Autodesk Inventor part; units mm, degrees
ref_plane "P3_XY" through (0, 0, 0) normal (0, 0, -1) x (1, 0, 0)
ref_plane "P3_YZ" through (0, 0, 0) normal (1, 0, 0) x (0, -1, 0)
ref_plane "P3_ZX" through (0, 0, 0) normal (0, -1, 0) x (0, 0, -1)
sketch "Sketch_1" plane through (0, 0, 0) normal (1, 0, 0) x (0, 0, -1)
  line L0 (0, 12.3912) -> (0, -11.05)
  line L1 (0, -11.05) -> (1, -11.05)
  line L2 (1, -11.05) -> (1, 12.4)
  line L3 (1, 12.4) -> (5.6693, 12.4)
  arc A0 (6.1684, 11.8695) -> (5.6693, 12.4) centre (5.6693, 11.9) ccw
  line L4 (6.1684, 11.8695) -> (4.8747, -9.2828)
  arc A1 (4.8747, -9.2828) -> (5.3282, -10.1825) centre (5.8728, -9.3439) ccw
  line L5 (5.3282, -10.1825) -> (7.9554, -11.8887)
  line L6 (7.9554, -11.8887) -> (8.5, -11.05)
  line L7 (8.5, -11.05) -> (6.1173, -9.5027)
  arc A2 (5.8906, -9.0528) -> (6.1173, -9.5027) centre (6.3897, -9.0834) ccw
  line L8 (5.8906, -9.0528) -> (7.1957, 12.2848)
  arc A3 (7.1957, 12.2848) -> (6.2063, 13.3458) centre (6.1975, 12.3459) ccw
  line L9 (6.2063, 13.3458) -> (1.0087, 13.3912)
  arc A4 (1.0087, 13.3912) -> (0, 12.3912) centre (1, 12.3912) ccw
extrude "Extrusion1" add sketch "Sketch_1" along normal mid plane 18
sketch "Sketch_2" plane through (0, 0, 0) normal (0, 0, 1) x (1, 0, 0)
  line L0 (-6.75, 16.5) -> (-6.75, 12.5)
  arc A0 (-6.75, 12.5) -> (-5.75, 11.5) centre (-5.75, 12.5) ccw
  line L1 (-5.75, 11.5) -> (5.75, 11.5)
  arc A1 (5.75, 11.5) -> (6.75, 12.5) centre (5.75, 12.5) ccw
  line L2 (6.75, 12.5) -> (6.75, 16.5)
  line L3 (6.75, 16.5) -> (-6.75, 16.5)
extrude "Extrusion2" cut sketch "Sketch_2" against normal blind 8
sketch "Sketch_3" plane through (0, 0, -1) normal (0, 0, 1) x (1, 0, 0)
  line L0 (-6.5, -12) -> (6.5, -12)
  line L1 (6.5, -12) -> (6.5, 13)
  line L2 (6.5, 13) -> (-6.5, 13)
  line L3 (-6.5, 13) -> (-6.5, -12)
extrude "Extrusion3" cut sketch "Sketch_3" against normal blind 8
sketch "Sketch_4" plane through (0, 0, 0) normal (1, 0, 0) x (0, 0, -1)
  arc A0 (4, -7.9626) -> (5.1384, -10.0593) centre (6.5, -7.9626) ccw
  line L0 (5.1384, -10.0593) -> (7.9554, -11.8887)
  line L1 (7.9554, -11.8887) -> (8.5, -11.05)
  line L2 (8.5, -11.05) -> (5.4554, -9.0728)
  arc A1 (5, -8.2341) -> (5.4554, -9.0728) centre (6, -8.2341) ccw
  line L3 (5, -8.2341) -> (5, 13.4)
  line L4 (5, 13.4) -> (4, 13.4)
  line L5 (4, 13.4) -> (4, -7.9626)
extrude "Extrusion4" add sketch "Sketch_4" along normal mid plane 13
sketch "Sketch_5" plane through (0, 0, 0) normal (1, 0, 0) x (0, 0, -1)
  line L0 (13, 0) -> (4, 0)
  line L1 (4, 0) -> (4, 5.7)
  line L2 (4, 5.7) -> (5, 5.7)
  arc A0 (5, 5.7) -> (6, 4.7) centre (6, 5.7) ccw
  line L3 (6, 4.7) -> (12, 4.7)
  arc A1 (13, 3.7) -> (12, 4.7) centre (12, 3.7) ccw
  line L4 (13, 3.7) -> (13, 0)
  line L5 (13, 0) -> (4, 0)
revolve "Revolution1" add sketch "Sketch_5" angle 360 about axis through (0, 0, -13) along (0, 0, -1)
sketch "Sketch6" plane through (0, 0, -13) normal (0, 0, -1) x (-1, 0, 0)
  point P0 (0, 0)
hole "Hole1" at (0, 0, -13) direction (0, 0, 1) diameter 7 depth 14
ref_plane "P3_XY" through (0, 0, 0) normal (0, 0, -1) x (1, 0, 0)
ref_plane "P3_YZ" through (0, 0, 0) normal (1, 0, 0) x (0, -1, 0)
ref_plane "P3_ZX" through (0, 0, 0) normal (0, -1, 0) x (0, 0, -1)
properties part number "8617.540_P3"
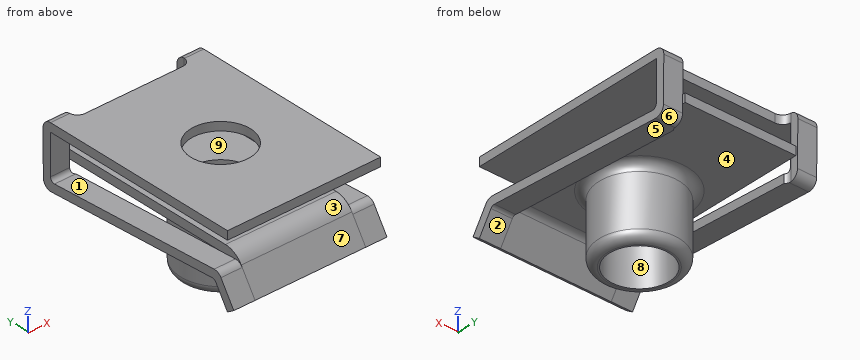
For this review, take the finished solid that the model builds, in its own axes (mm). Face numbers are marked on the shaded views. A direction names the side the tool comes from. Round coordinates to 2 decimals unless told otherwise and drop trailing zeros. Order: outer loops, then holes, each group sorted by start corner. A loop starts at its lowest first (then second) coordinate and runs counter-clockwise, first axis right, second up. Notation, with made-up numbers: M -11.5,12 L 30.5,12 A27 cw 30.5,32 Z; hole C -21.5,-6.5 d8. An arc over 180 degrees is marked long. Use a Markdown table: item, result. Add a question column.
Item 1: Add section D-D, the plane y = 0. State how many separate pieces and enclosed holes the cut face has, then the cut area to 3 significant figures.
Item 2: Add section B-B, the plane y = -6. Give the boundary of the cut face in (x, z).
Item 3: Mouldability with a two-part tool opening along Z and no side actions: class the marked faces 6, 7, 8 and 9 as released by +Z, released by -Z, zero draft, split by the parting line, or undercut.
Item 4: Insertion check: pin 1 (0.7 mm diameter, centred on x = 8, z = -2.5, fed in from -Y); pin 2 (0.8 mm diameter, centred on x = 0, z = -0.5, fed in from +Y); pin 3 (1 mm diameter, centred on y = 4.5, z = -4.5, fed in from -X). Each pin has a flat end and moves straight along its axis. Give the tip position at first contact, or say it passes through.
Item 5: Add section A-A, the plane x = 0. Give the boundary of the cut face in (y, z).
Item 6: To check wall thickness, follow line 1 along X through (y, z) = (0, -6.25); line 2 along X through (y, z) = (0, -0.7); line 3 along Y through (x, z) = (-1.25, -5.75). State the ranges of each line that lie inside material, in increasing order.
Item 7: Tool access review of the marked faces 1, 2, 3, 4 and 5: name each direction out of +Z, -Z, +X, -X, +Y, -Y from which nothing blocks a thin tool from reaching the whole face with its end or side.
Item 8: Add section C-C, the plane z = -11. Give the boundary of the cut face in (x, y).
Geometry results:
| question | item | result |
|---|---|---|
| 1 | separate pieces | 6 |
| 1 | enclosed holes | 0 |
| 1 | area | 41.2 mm² |
| 2 | outline | M -9,-6.08 L -6.5,-6.08 L -6.5,-5.08 L -9,-5.08 Z; M -9,-1 L 9,-1 L 9,0 L -9,0 Z; M -6.5,-5 L 6.5,-5 L 6.5,-4 L -6.5,-4 Z; M 6.5,-6.08 L 9,-6.08 L 9,-5.08 L 6.5,-5.08 Z |
| 3 | face 6 | released by -Z |
| 3 | face 7 | undercut |
| 3 | face 8 | zero draft |
| 3 | face 9 | undercut |
| 4 | pin 1 | stops at y = 12.4 |
| 4 | pin 2 | stops at y = 11.5 |
| 4 | pin 3 | stops at x = -6.5 |
| 5 | outline | M -11.89,-7.96 L -11.05,-8.5 L -9.07,-5.46 A1 cw -8.23,-5 L -5.7,-5 A1 cw -4.7,-6 L -4.7,-12 A1 ccw -3.7,-13 L -3.5,-13 L -3.5,-4 L -7.96,-4 A2.5 ccw -10.06,-5.14 Z; M -11.05,-1 L -3.5,-1 L -3.5,0 L -11.05,0 Z; M 3.5,-13 L 3.7,-13 A1 ccw 4.7,-12 L 4.7,-6 A1 cw 5.7,-5 L 13.4,-5 L 13.4,-4 L 3.5,-4 Z; M 3.5,-1 L 11.5,-1 L 11.5,0 L 3.5,0 Z |
| 6 | line 1 | x = -9 to -6.5, -4.7 to -3.5, 3.5 to 4.7, 6.5 to 9 |
| 6 | line 2 | x = -9 to -3.5, 3.5 to 9 |
| 6 | line 3 | y = -10.46 to -9.26, -4.56 to -3.27, 3.27 to 4.56 |
| 7 | face 1 | -X |
| 7 | face 2 | -Z, +X, -X |
| 7 | face 3 | +X, -X, -Y |
| 7 | face 4 | -Z |
| 7 | face 5 | -Z, +X |
| 8 | outline | C 0,0 d9.4; hole C 0,0 d7 |
